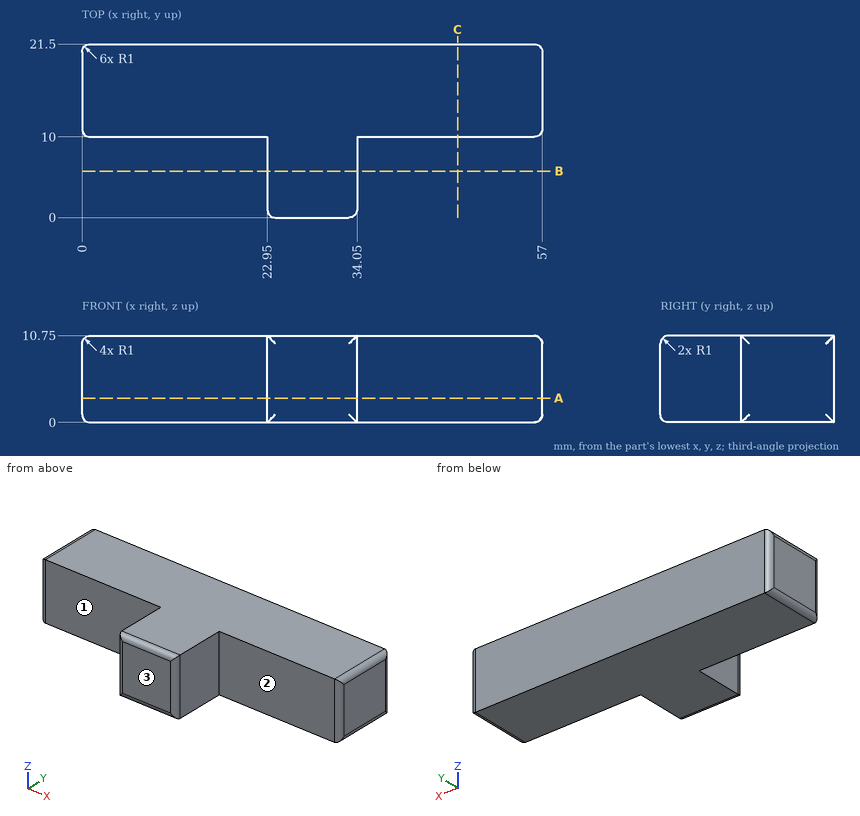
Could you check a few things on this drawing? It's one solid part, dimensions in mm from its lowest x, y, z. A direction names the side the tool comes from. Coordinates: 2 decimals unless noted, no trailing zeros. Order: outer loops, then holes, each group sorted by start corner. A loop starts at its lowest first (then second) coordinate and runs counter-clockwise, first axis right, second up. Notation, with made-up numbers: (39.5, 1) - (63.5, 1) arc R36 cw to (63.5, 36) - close; hole circle Ø8 at (15, -40). An arc over 180 degrees is marked (long way). One line per question, with ' | ' between items.
(1) Will these pins go through, and if not, where does the flat tip stop? pin 1 (4.5 mm diameter, centred on y = 6, z = 5, fed in from -X); pin 2 (4 mm diameter, centred on y = 6, z = 6, fed in from +X); pin 3 (3 mm diameter, centred on x = 47.5, z = 7, fed in from -Y).
Report:
pin 1: stops at x = 22.95 | pin 2: stops at x = 34.05 | pin 3: stops at y = 10
(2) For the marked faces 1, 2 and 3, which set-ups out of +Z, -Z, +X, -X, +Y, -Y let a thin tool reach every point of the face, with its end or its side?
Report:
face 1: +Z, -Z, -X, -Y | face 2: +Z, -Z, +X, -Y | face 3: +Z, -Z, +X, -X, -Y
(3) Suppose I cut it at C-C on x = 46.5. List the corners of the cut face in (y, z) for me, and give its area (3 significant figures).
Report:
outline: (10, 0) - (21.5, 0) - (21.5, 10.75) - (10, 10.75) - close | area: 124 mm2
(4) Suppose I cut it at A-A on z = 3. List the corners of the cut face in (x, y) for me, and give its area (3 significant figures).
Report:
outline: (0, 11) arc R1 ccw to (1, 10) - (22.95, 10) - (22.95, 1) arc R1 ccw to (23.95, 0) - (33.05, 0) arc R1 ccw to (34.05, 1) - (34.05, 10) - (56, 10) arc R1 ccw to (57, 11) - (57, 20.5) arc R1 ccw to (56, 21.5) - (1, 21.5) arc R1 ccw to (0, 20.5) - close | area: 765 mm2
(5) Suppose I cut it at B-B on y = 5.75. List the corners of the cut face in (x, z) for me, and give its area (3 significant figures).
Report:
outline: (22.95, 0) - (34.05, 0) - (34.05, 10.75) - (22.95, 10.75) - close | area: 119 mm2
(6) If I drill on L1, parallel to X at y = 2.25, z = 7; L2, parallel to Y at x = 47, z = 8.5, over which ranges is the centre line in solid material (lowest first)?
Report:
L1: x = 22.95 to 34.05 | L2: y = 10 to 21.5
